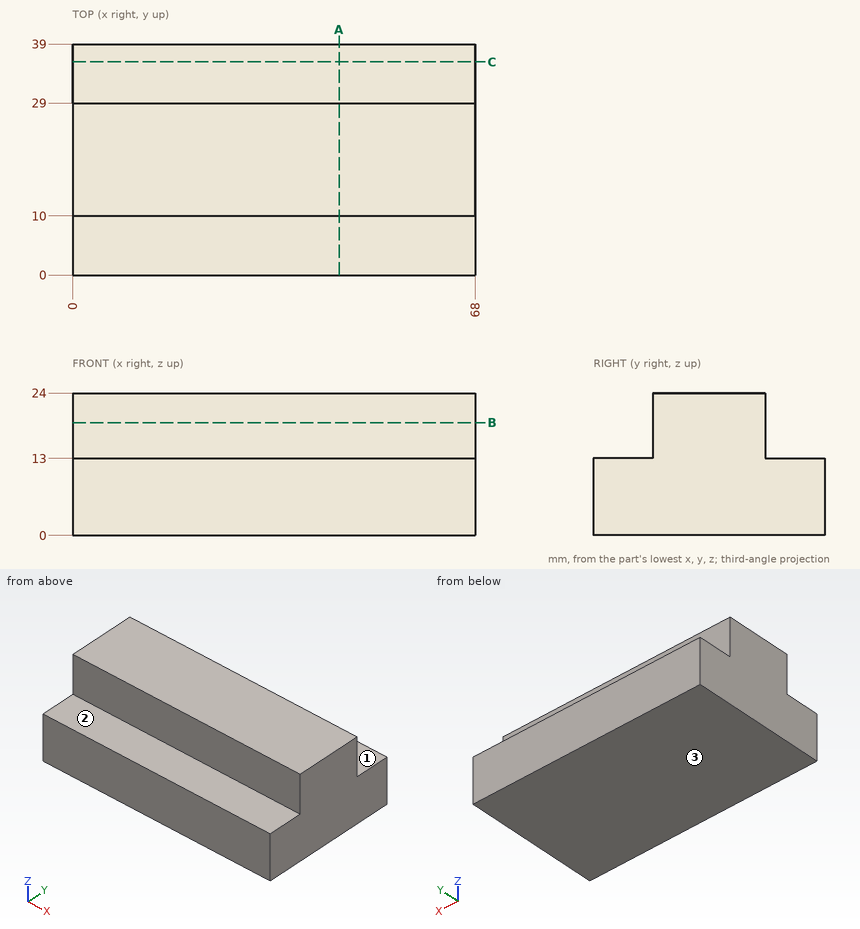
Design review of the part shown in the three views and the two pictorial views. Dimensions are in mm from the part's minimum x, y and z. A direction names the side the tool comes from. Round coordinates to 2 decimals unless told otherwise and drop trailing zeros. Order: outer loops, then holes, each group sorted by start corner. A loop starts at its lowest first (then second) coordinate and runs counter-clockwise, first axis right, second up.
(1) For P1, Ø9, axis at x = 43, z = 18.5, coming from the +Y side; P2, Ø1.5, axis at x = 28.5, z = 18, coming from the -Y side; P3, Ø5, axis at x = 23, y = 5.5, coming from the +Z side, all flat-tipped, find the tip position at first contact; note any pin that passes through.
Working result:
P1: stops at y = 29
P2: stops at y = 10
P3: stops at z = 13
(2) Wall thickness on L1, parallel to Y at x = 48, z = 13.75; L2, parallel to Z at x = 52, y = 29.5: over which ranges is each line inside the solid? List them lowest first.
Working result:
L1: y = 10 to 29
L2: z = 0 to 13
(3) Take a section at A-A, the plane x = 45. State the section outline as (y, z) points, plus the area to 3 significant figures.
Working result:
outline: (0, 0) - (39, 0) - (39, 13) - (29, 13) - (29, 24) - (10, 24) - (10, 13) - (0, 13) - close
area: 716 mm2
(4) Take a section at B-B, the plane z = 19. State the section outline as (x, y) points, plus the area to 3 significant figures.
Working result:
outline: (0, 10) - (68, 10) - (68, 29) - (0, 29) - close
area: 1,290 mm2
(5) Tool access review of the marked faces 1, 2 and 3: name each direction out of +Z, -Z, +X, -X, +Y, -Y from which nothing blocks a thin tool from reaching the whole face with its end or side.
Working result:
face 1: +Z, +X, -X, +Y
face 2: +Z, +X, -X, -Y
face 3: -Z, +X, -X, +Y, -Y
(6) Take a section at C-C, the plane y = 36. State the section outline as (x, z) points.
Working result:
outline: (0, 0) - (68, 0) - (68, 13) - (0, 13) - close
